Geometry: final body of the model. Coordinates: model frame, mm. A direction names the side the tool comes from. Round coordinates to 2 decimals unless told otherwise and drop trailing zeros. Loops run counter-clockwise (first coordinate to the right, second up) from the corner with the lowest first, then second, coordinate; pieces in that order, holes last. Notation, with made-up numbers: M 38,24.25 L 43,24.25 A13 ccw 43,42.25 Z; hole C 69,6.5 d7. An arc over 180 degrees is marked long. Answer as a JSON object with one key per item and string values.
from build123d import *

# Parameters (mm, degrees)
F0_W          = 80
F0_H          = 90
F1_DEPTH      = 60
F1_DEPTH_BACK = 60
F2_R          = 39.99999
F3_R          = 16
F4_DEPTH      = 120.001
F5_W          = 80
F5_H          = 64.99999
F5_H_2        = 35.00001
F6_DEPTH      = 80.001
F7_R          = 7.5
F8_DEPTH      = 90.001
F7_R_2        = 30
F9_DEPTH      = 5
F10_DEPTH     = 20


# Not quite as in the source:
# - a fillet or chamfer is up to 0.001 mm smaller than in the source, because OpenCascade refuses the exact size


with BuildPart() as f1:
    # F0 (on Front) → F1 (new body, two sides)
    with BuildSketch(Plane.XZ) as f1_sk:
        Rectangle(F0_W, F0_H)
    extrude(amount=F1_DEPTH)
    extrude(f1_sk.sketch, amount=-F1_DEPTH_BACK)

    # F2 (radius 40 in the source; OpenCascade refuses exactly that, so slightly less here)
    f2_edges = [f1.edges().sort_by_distance(p)[0] for p in [
        (40, 0, -45),
        (-40, 0, -45),
    ]]
    fillet(f2_edges, radius=F2_R)

    # F3 (on face) → F4 (cut, through all)
    with BuildSketch(Plane.XZ.offset(60)):
        Circle(F3_R)
    extrude(amount=-F4_DEPTH, mode=Mode.SUBTRACT)

    # F5 (on face) → F6 (cut, through all)
    with BuildSketch(Plane(origin=(-40, 0, 0), x_dir=(0, -1, 0), z_dir=(-1, 0, 0))):
        with Locations((0, -37.500005)):
            Rectangle(F5_W, F5_H)
        with Locations((0, 12.499995)):
            Rectangle(F5_W, F5_H_2)
    extrude(amount=-F6_DEPTH, mode=Mode.SUBTRACT)

    # F7 (on face) → F8 (cut, through all)
    with BuildSketch(Plane.XY.offset(45)):
        Circle(F7_R)
    extrude(amount=-F8_DEPTH, mode=Mode.SUBTRACT)

    # F7 (on face) → F9 (join)
    with BuildSketch(Plane.XY.offset(45)):
        Circle(F7_R_2)
        Circle(F7_R, mode=Mode.SUBTRACT)
    extrude(amount=F9_DEPTH)

    # F7 (on face) → F10 (join)
    with BuildSketch(Plane.XY.offset(45)):
        with BuildLine():
            ThreePointArc((-40, 0), (0, -40), (40, 0))
            ThreePointArc((40, 0), (0, 40), (-40, 0))
        make_face()
        Circle(F7_R_2, mode=Mode.SUBTRACT)
    extrude(amount=F10_DEPTH)


solid = f1.part
1) Reachability of faces 1 (the cylindrical face through (-29.97, 1.32, 57.4)), 2 (the flat face through (-1, 43, 45)), 3 (the flat face through (-1, -44, 45)), 4 (the flat face through (-1, -8, 30)) from +Z, -Z, +X, -X, +Y, -Y: full face, straight path, thin tool, end or side. Return the list, or none.
Results:
{"face 1": "+Z", "face 2": "+Z, +Y", "face 3": "+Z, -Y", "face 4": "-Z, +X, -X"}
2) Section query D-D (z = -18). Return the cut outline in (x, y).
Results:
{"outline": "M -37.83,-60 L 37.83,-60 L 37.83,-40 L -37.83,-40 Z; M -37.83,40 L 37.83,40 L 37.83,60 L -37.83,60 Z"}
3) Section query A-A (z = 0). Return the cut outline in (x, y).
Results:
{"outline": "M -40,-60 L -16,-60 L -16,-40 L -40,-40 Z; M -40,40 L -16,40 L -16,60 L -40,60 Z; M 16,-60 L 40,-60 L 40,-40 L 16,-40 Z; M 16,40 L 40,40 L 40,60 L 16,60 Z"}
4) Ray query, line 1 (Y direction, x = -0.5, z = 32.5); line 2 (Y direction, x = -7.5, z = -30.5); line 3 (Z direction, x = 1.5, y = -29.5). Return the intervals inside material, ascending.
Results:
{"line 1": "-60 to -7.48, 7.48 to 60", "line 2": "-60 to -40, 40 to 60", "line 3": "30 to 50"}
5) Section query B-B (y = 38). Return the cut outline in (x, z).
Results:
{"outline": "M -40,30 L 40,30 L 40,45 L 12.49,45 L 12.49,65 L -12.49,65 L -12.49,45 L -40,45 Z"}
6) Pull-direction query (Y, two-part tool) for faces 5 (the cylindrical face through (28.594, 49.86, -32.972)), 6 (the flat face through (6, -6, 50)), 7 (the cylindrical face through (-32, -24, 55)); classes: +Y half, -Y half, draft (parallel to the pull), parting line (faces both ways), or undercut.
Results:
{"face 5": "draft", "face 6": "undercut", "face 7": "parting line"}
7) Section query C-C (x = -19). Return the cut outline in (y, z).
Results:
{"outline": "M -60,-40.2 L -40,-40.2 L -40,30 L 40,30 L 40,-40.2 L 60,-40.2 L 60,45 L 35.2,45 L 35.2,65 L 23.22,65 L 23.22,50 L -23.22,50 L -23.22,65 L -35.2,65 L -35.2,45 L -60,45 Z"}
8) Pin query (flat end, axial travel): P1, Ø5, axis at x = 29.5, y = 48, coming from the +Z side; P2, Ø1, axis at x = 21.5, y = 19, coming from the +Z side; P3, Ø2, axis at y = 40, z = -19, coming from the +X side. Return the tip coordinate at first contact, or that it passes through.
Results:
{"P1": "z = 45", "P2": "z = 50", "P3": "x = 37.83"}
